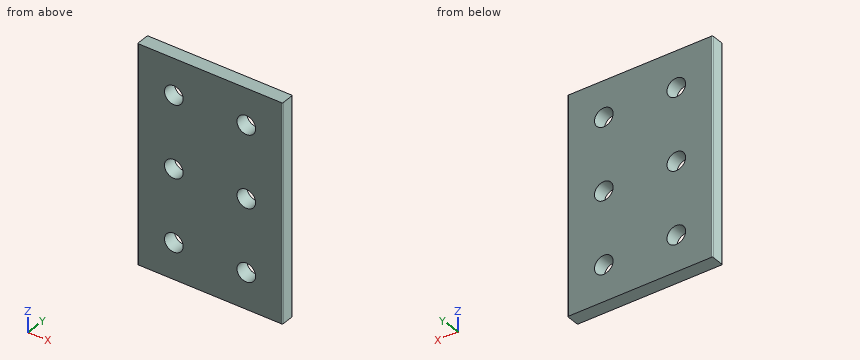
from build123d import *

# Parameters (mm, degrees)
BOSS_EXTRUDE1_OUTLINE_W  = 4.7752
BOSS_EXTRUDE1_OUTLINE_H  = 76.2
BOSS_EXTRUDE1_DEPTH      = 50.8
F_0_257_DIAMETER_HOLE1_D = 6.5278
FILLET1_R                = 0.381
LPATTERN1_COUNT          = 4
LPATTERN1_PITCH          = 25.4
LPATTERN1_COUNT_DIR2     = 2
LPATTERN1_PITCH_DIR2     = 25.4


# Read off the part's stored shape, not the designer's step: Boss-Extrude1
with BuildPart() as part:
    # Boss-Extrude1 outline → Boss-Extrude1 (new body)
    with BuildSketch(Plane.YZ):
        with Locations((2.3876, 38.1)):
            Rectangle(BOSS_EXTRUDE1_OUTLINE_W, BOSS_EXTRUDE1_OUTLINE_H)
    extrude(amount=BOSS_EXTRUDE1_DEPTH)

    # F (0.257) Diameter Hole1 (through all)
    with Locations(Plane(origin=(0, 4.7752, 0), x_dir=(-1, 0, 0), z_dir=(0, 1, 0))):
        with Locations((-38.1, 63.5)):
            f_0_257_diameter_hole1 = Hole(F_0_257_DIAMETER_HOLE1_D / 2)

    # Fillet1
    fillet1_edges = [part.edges().sort_by_distance(p)[0] for p in [
        (50.8, 4.7752, 38.1),
        (0, 4.7752, 38.1),
        (50.8, 0, 38.1),
        (0, 0, 38.1),
    ]]
    fillet(fillet1_edges, radius=FILLET1_R)

    # LPattern1: F _0.257_ Diameter Hole1 4 × 2
    with Locations(*[(-j * LPATTERN1_PITCH_DIR2, 0, -i * LPATTERN1_PITCH) for i in range(LPATTERN1_COUNT) for j in range(LPATTERN1_COUNT_DIR2) if (i, j) != (0, 0)]):
        add(f_0_257_diameter_hole1, mode=Mode.SUBTRACT)


solid = part.part
For this review, take the finished solid that the model builds, in its own axes (mm). Give positions to 0.01 mm unless a question says otherwise; leave off trailing zeros. Order: outer loops, then holes, each group sorted by start corner. A loop starts at its lowest first (then second) coordinate and runs counter-clockwise, first axis right, second up. Notation, with made-up numbers: (12.25, 74.25) - (58.25, 74.25) arc R12 ccw to (58.25, 79.25) - close; hole circle Ø4 at (-16.75, 86). An arc over 180 degrees is marked (long way). Answer as a JSON object with one key per item and string values. Group by question number.
Item 1: Take a section at A-A on x = 38.1. Give the boundary of the cut face in (y, z), and give its area (3 significant figures).
Item 2: Take a section at B-B on z = 63.5. Give the boundary of the cut face in (x, y), and give its area (3 significant figures).
Item 3: Wall thickness on line 1 along Z through (x, y) = (38.1, 1.8); line 2 along X through (y, z) = (1.75, 12.5); line 3 along Z through (x, y) = (14.5, 4.1): over which ranges is each line inside the solid? List them lowest first.
Item 4: Take a section at C-C on y = 1.65. Give the boundary of the cut face in (x, z).
Reported:
{
 "1": {"outline": "(0, 0) - (4.78, 0) - (4.78, 9.44) - (0, 9.44) - close; (0, 15.96) - (4.78, 15.96) - (4.78, 34.84) - (0, 34.84) - close; (0, 41.36) - (4.78, 41.36) - (4.78, 60.24) - (0, 60.24) - close; (0, 66.76) - (4.78, 66.76) - (4.78, 76.2) - (0, 76.2) - close", "area": "270 mm^2"},
 "2": {"outline": "(0, 0.38) arc R0.38 ccw to (0.38, 0) - (9.44, 0) - (9.44, 4.78) - (0.38, 4.78) arc R0.38 ccw to (0, 4.39) - close; (15.96, 0) - (34.84, 0) - (34.84, 4.78) - (15.96, 4.78) - close; (41.36, 0) - (50.42, 0) arc R0.38 ccw to (50.8, 0.38) - (50.8, 4.39) arc R0.38 ccw to (50.42, 4.78) - (41.36, 4.78) - close", "area": "180 mm^2"},
 "3": {"line 1": "0 to 9.44, 15.96 to 34.84, 41.36 to 60.24, 66.76 to 76.2", "line 2": "0 to 9.44, 15.96 to 34.84, 41.36 to 50.8", "line 3": "0 to 9.98, 15.42 to 35.38, 40.82 to 60.78, 66.22 to 76.2"},
 "4": {"outline": "(0, 0) - (50.8, 0) - (50.8, 76.2) - (0, 76.2) - close; hole circle Ø6.53 at (12.7, 12.7); hole circle Ø6.53 at (12.7, 38.1); hole circle Ø6.53 at (12.7, 63.5); hole circle Ø6.53 at (38.1, 12.7); hole circle Ø6.53 at (38.1, 38.1); hole circle Ø6.53 at (38.1, 63.5)"}
}
